The listing builds one solid part. Answer for the finished solid, in the listing's coordinates (mm). A direction names the side the tool comes from. Coordinates: 2 decimals unless noted, no trailing zeros. Order: outer loops, then holes, each group sorted by start corner. A loop starts at its lowest first (then second) coordinate and runs counter-clockwise, first axis right, second up. Notation, with made-up numbers: (45.25, 70) -> (98.25, 70) arc R16 cw to (98.25, 75) -> close; hole circle Ø8 at (39.5, 47.5). An arc over 180 degrees is marked (long way). Return JSON: item names as keys, results as strings.
Autodesk Inventor part; units mm, degrees
ref_plane "YZ Plane" through (0, 0, 0) normal (1, 0, 0) x (0, 1, 0)
ref_plane "XZ Plane" through (0, 0, 0) normal (0, 1, 0) x (-1, 0, 0)
ref_plane "XY Plane" through (0, 0, 0) normal (0, 0, 1) x (1, 0, 0)
sketch "スケッチ1" plane through (0, 0, 0) normal (0, 0, 1) x (1, 0, 0)
  circle A0 centre (-35.9404, 22.842) radius 1.5
  circle A1 centre (5.9362, 53.5882) radius 1.5
  circle A2 centre (127.6431, 30.2622) radius 1.5
  line L0 (22.1499, 50.4807) -> (113.9448, 32.8876)
  circle A3 centre (5.9362, 53.5882) radius 4.5
  circle A4 centre (127.6431, 30.2622) radius 4.5
  circle A5 centre (-35.9404, 22.842) radius 3
  line L1 (5.0892, 49.1686) -> (11.145, 48.008)
  line L2 (11.145, 48.008) -> (22.1499, 50.4807)
  line L3 (113.9448, 32.8876) -> (122.4523, 26.6751)
  line L4 (122.4523, 26.6751) -> (126.7961, 25.8426)
  line L5 (4.4419, 57.8328) -> (15.2047, 61.622)
  line L6 (-37.785, 25.2079) -> (3.1694, 57.1371)
  line L7 (3.5126, 49.7966) -> (-34.0959, 20.4761)
  line L8 (122.0018, 41.1536) -> (130.601, 33.6535)
  circle A6 centre (80.3181, 36.2778) radius 3
  circle A7 centre (80.3181, 36.2778) radius 4.5
  line L9 (128.2106, 34.7263) -> (80.8855, 40.7419)
  circle A8 centre (80.4743, 23.124) radius 1.5
  line L10 (120.4636, 35.711) -> (121.0283, 38.6574)
  line L11 (15.1864, 58.9428) -> (14.6217, 55.9964)
  circle A9 centre (66.9779, 42.9073) radius 1.5
  circle A10 centre (66.9779, 42.9073) radius 3
  line L12 (29.9182, 56.1193) -> (29.3535, 53.1729)
  arc A11 (17.2488, 58.5475) -> (15.1864, 58.9428) centre (16.2176, 58.7451) ccw
  arc A12 (29.9182, 56.1193) -> (27.8558, 56.5146) centre (28.887, 56.3169) ccw
  arc A13 (27.2911, 53.5682) -> (29.3535, 53.1729) centre (28.3223, 53.3705) ccw
  arc A14 (14.6217, 55.9964) -> (16.6841, 55.6011) centre (15.6529, 55.7987) ccw
  line L13 (17.2488, 58.5475) -> (27.8558, 56.5146)
  line L14 (16.6841, 55.6011) -> (27.2911, 53.5682)
  arc A15 (31.8825, 55.7428) -> (27.0019, 58.7146) centre (28.887, 56.3169) ccw
  line L15 (27.0019, 58.7146) -> (18.8556, 60.2759)
  arc A16 (18.8556, 60.2759) -> (15.2047, 61.622) centre (16.2176, 58.7451) ccw
  line L16 (106.2964, 41.4808) -> (105.7317, 38.5345)
  arc A17 (108.3589, 41.0856) -> (106.2964, 41.4808) centre (107.3276, 41.2832) ccw
  arc A18 (121.0283, 38.6574) -> (118.9658, 39.0527) centre (119.997, 38.855) ccw
  arc A19 (118.4011, 36.1063) -> (120.4636, 35.711) centre (119.4323, 35.9086) ccw
  arc A20 (105.7317, 38.5345) -> (107.7942, 38.1392) centre (106.7629, 38.3368) ccw
  line L17 (31.8825, 55.7428) -> (104.3322, 41.8573)
  line L18 (108.3589, 41.0856) -> (118.9658, 39.0527)
  line L19 (107.7942, 38.1392) -> (118.4011, 36.1063)
  arc A21 (122.0018, 41.1536) -> (118.1119, 41.2527) centre (119.997, 38.855) ccw
  line L20 (118.1119, 41.2527) -> (109.9656, 42.814)
  arc A22 (109.9656, 42.814) -> (104.3322, 41.8573) centre (107.3276, 41.2832) ccw
  line L21 (30.3885, 58.9717) -> (38.2584, 54.5208)
  line L22 (16.7917, 61.7406) -> (29.4611, 59.3124)
  line L23 (120.5711, 41.8505) -> (107.9017, 44.2787)
  line L24 (106.8479, 44.2952) -> (98.5267, 42.97)
  point P0 (0, 0)
  point P1 (0, 0)
  point P2 (0, 0)
  dimension "d53" = 9
  dimension "d49" = 9
  dimension "d50" = 9
  dimension "d51" = 6
  dimension "d52" = 6
  dimension "d54" = 47.7059
  dimension "d55" = 47.7059
  dimension "d56" = 3
  dimension "d57" = 3
  dimension "d58" = 8.0769
  dimension "d59" = 8.0769
  dimension "d60" = 3
  dimension "d61" = 6
  dimension "d62" = 61.9691
  dimension "d63" = 61.9691
  dimension "d64" = 15
  dimension "d65" = 2.1
  dimension "d66" = 2
  dimension "d67" = 2
  dimension "d68" = 2
  dimension "d69" = 15
  dimension "d70" = 2.1
  dimension "d71" = 7
  dimension "d72" = 2
  dimension "d73" = 2
sketch "スケッチ2" plane through (0, 0, 0) normal (0, 0, 1) x (1, 0, 0)
  line L0 (17.1, 0) -> (90.6683, 0)
  line L1 (107.7683, 0) -> (107.7683, -47)
  line L2 (90.6683, -47) -> (17.1, -47)
  line L3 (0, -47) -> (0, 0)
  line L4 (0, 0) -> (0, 3)
  line L5 (0, 3) -> (15, 3)
  line L6 (15, 3) -> (15, 0)
  line L7 (107.7683, 0) -> (107.7683, 3)
  line L8 (107.7683, 3) -> (92.7683, 3)
  line L9 (92.7683, 3) -> (92.7683, 0)
  line L10 (107.7683, -47) -> (107.7683, -50)
  line L11 (107.7683, -50) -> (92.7683, -50)
  line L12 (92.7683, -50) -> (92.7683, -47)
  line L13 (0, -47) -> (0, -50)
  line L14 (0, -50) -> (15, -50)
  line L15 (15, -50) -> (15, -47)
  arc A0 (15, 0) -> (17.1, 0) centre (16.05, 0) ccw
  arc A1 (90.6683, 0) -> (92.7683, 0) centre (91.7183, 0) ccw
  arc A2 (92.7683, -47) -> (90.6683, -47) centre (91.7183, -47) ccw
  arc A3 (17.1, -47) -> (15, -47) centre (16.05, -47) ccw
  line L16 (15.1864, 58.9428) -> (14.6217, 55.9964)
  line L17 (120.4636, 35.711) -> (121.0283, 38.6574)
  dimension "d30" = 107.7683
  dimension "d31" = 47
  dimension "d32" = 3
  dimension "d33" = 15
  dimension "d34" = 3
  dimension "d35" = 15
  dimension "d36" = 3
  dimension "d37" = 15
  dimension "d38" = 3
  dimension "d39" = 3
  dimension "d40" = 15
  dimension "d41" = 2.1
  dimension "d42" = 2.1
  dimension "d43" = 2.1
  dimension "d44" = 2.1
  dimension "d45" = 3
  dimension "d46" = 3
  dimension "d74" = 107.7683
extrude "押し出し1" add sketch "スケッチ2" along normal blind 3
sketch "スケッチ3" plane through (0, 0, 0) normal (0, 0, -1) x (-1, 0, 0)
  line L0 (0, 3) -> (0, -50)
  line L1 (-15, 3) -> (0, 3)
  line L2 (-15, 0) -> (-15, 3)
  arc A0 (-17.1, 0) -> (-15, 0) centre (-16.05, 0) ccw
  line L3 (-90.6683, 0) -> (-17.1, 0)
  arc A1 (-92.7683, 0) -> (-90.6683, 0) centre (-91.7183, 0) ccw
  line L4 (-92.7683, 3) -> (-92.7683, 0)
  line L5 (-107.7683, 3) -> (-92.7683, 3)
  line L6 (-107.7683, -50) -> (-107.7683, 3)
  line L7 (-92.7683, -50) -> (-107.7683, -50)
  line L8 (-92.7683, -47) -> (-92.7683, -50)
  arc A2 (-90.6683, -47) -> (-92.7683, -47) centre (-91.7183, -47) ccw
  line L9 (-17.1, -47) -> (-90.6683, -47)
  arc A3 (-15, -47) -> (-17.1, -47) centre (-16.05, -47) ccw
  line L10 (-15, -50) -> (-15, -47)
  line L11 (0, -50) -> (-15, -50)
  line L12 (-104.7683, -3) -> (-3, -3)
  line L13 (-3, -3) -> (-3, -44)
  line L14 (-3, -44) -> (-104.7683, -44)
  line L15 (-104.7683, -44) -> (-104.7683, -3)
  line L16 (-104.7683, -3) -> (-3, -44) construction
  arc A4 (-104.2078, -1.6087) -> (-106.2683, -3) centre (-104.7683, -3) ccw
  arc A5 (-3.5605, -45.3913) -> (-2.4395, -42.6087) centre (-3, -44) ccw
  line L17 (-3, -3) -> (-104.7683, -44) construction
  arc A6 (-2.4395, -4.3913) -> (-3.5605, -1.6087) centre (-3, -3) ccw
  arc A7 (-105.3288, -42.6087) -> (-104.2078, -45.3913) centre (-104.7683, -44) ccw
  line L18 (-3, -42.3828) -> (-49.8701, -23.5)
  line L19 (-53.8842, -21.8828) -> (-100.7543, -3)
  line L20 (-100.7543, -44) -> (-53.8842, -25.1172)
  line L21 (-49.8701, -23.5) -> (-3, -4.6172)
  line L22 (-104.7683, -4.6172) -> (-57.8982, -23.5)
  line L23 (-53.8842, -25.1172) -> (-7.014, -44)
  line L24 (-7.014, -3) -> (-53.8842, -21.8828)
  line L25 (-57.8982, -23.5) -> (-104.7683, -42.3828)
  point P0 (0, 0)
  point P1 (-53.8842, -23.5)
  point P2 (-53.8842, -23.5)
  dimension "d75" = 3
  dimension "d76" = 3
  dimension "d77" = 3
  dimension "d78" = 3
  dimension "d79" = 3
  dimension "d80" = 3
extrude "押し出し2" cut sketch "スケッチ3" against normal blind 2.5 contours L12 L24 L19 | L22 L25 L15 | L13 L18 L21 | L20 L23 L14
fillet "フィレット1" radius 1 12 edges at (100.7543, -3, 1.25) (104.7683, -4.6172, 1.25) (104.7683, -42.3828, 1.25) (100.7543, -44, 1.25) (57.8982, -23.5, 1.25) (53.8842, -21.8828, 1.25) (53.8842, -25.1172, 1.25) (49.8701, -23.5, 1.25) (7.014, -44, 1.25) (3, -42.3828, 1.25) (3, -4.6172, 1.25) (7.014, -3, 1.25)
equation "\"d55\" = d54"
equation "\"d59\" = d58"
equation "\"d63\" = d62"
equation "\"d30\" = d74"
properties part number "台形サスバー板" material "ポリカーボネート、クリア"
Item 1: Determine the mould class of faces 1 (the flat face through (92.768, 2, 1)), 2 (the cylindrical face through (91.7, -45.95, 1.48)), 3 (the flat face through (82.1, -13.75, 1.23)) for opening direction Y: pulls with the +Y half, pulls with the -Y half, needs draft (parallel to the pull), parting line crosses it, or undercut.
Answer list:
{"face 1": "needs draft", "face 2": "pulls with the -Y half", "face 3": "undercut"}
Item 2: Flat-ended cylindrical pins translate along their axes: pin 1 (1.5 mm diameter, centred on x = 60.5, z = 2, fed in from +Y); pin 2 (1.5 mm diameter, centred on x = 39.5, z = 2, fed in from -Y); pin 3 (5 mm diameter, centred on x = 65, y = -7, fed in from -Z). Find the tip coordinate at first contact, or state that the pin passes through.
Answer list:
{"pin 1": "y = 0", "pin 2": "y = -47", "pin 3": "z = 2.5"}
Item 3: Which of the six approach directions +Z, -Z, +X, -X, +Y, -Y give full straight-line access (tool end or side, diameter ignored) to faces 4 (the cylindrical face through (16.07, -1.05, 1.48)), 5 (the flat face through (15, -49, 1)), 6 (the cylindrical face through (11.187, -43.171, 1.268))?
Answer list:
{"face 4": "+Z, -Z, +Y", "face 5": "+Z, -Z, -Y", "face 6": "-Z"}
Item 4: The part is cut by section B-B on z = 1.05. Count the separate pieces of the cut face and the enclosed holes in it, plus the area to 3 significant figures.
Answer list:
{"separate pieces": "1", "enclosed holes": "4", "area": "1,720 mm2"}
Item 5: The part is cut by section D-D on x = 50.5. Determine the outline of the cut face in (y, z).
Answer list:
{"outline": "(-47, 0) -> (-44, 0) -> (-44, 2.5) -> (-26.48, 2.5) -> (-26.48, 0) -> (-20.52, 0) -> (-20.52, 2.5) -> (-3, 2.5) -> (-3, 0) -> (0, 0) -> (0, 3) -> (-47, 3) -> close"}
Item 6: The part is cut by section A-A on x = 16. Determine the outline of the cut face in (y, z).
Answer list:
{"outline": "(-45.95, 0) -> (-44, 0) -> (-44, 2.5) -> (-40.38, 2.5) -> (-40.38, 0) -> (-37.15, 0) -> (-37.15, 2.5) -> (-9.85, 2.5) -> (-9.85, 0) -> (-6.62, 0) -> (-6.62, 2.5) -> (-3, 2.5) -> (-3, 0) -> (-1.05, 0) -> (-1.05, 3) -> (-45.95, 3) -> close"}
Item 7: Find the intervals of material crossed by probe 1 along X at (y, z) = (-14, 1); probe 2 along Y at (x, z) = (58, 0.5); probe 3 along Y at (x, z) = (59, 0.95), in increasing order.
Answer list:
{"probe 1": "0 to 3, 26.29 to 34.32, 73.45 to 81.48, 104.77 to 107.77", "probe 2": "-47 to -44, -26.78 to -20.22, -3 to 0", "probe 3": "-47 to -44, -27.18 to -19.82, -3 to 0"}
Item 8: The part is cut by section C-C on y = -18. Determine the outline of the cut face in (x, z).
Answer list:
{"outline": "(0, 0) -> (3, 0) -> (3, 2.5) -> (36.22, 2.5) -> (36.22, 0) -> (44.25, 0) -> (44.25, 2.5) -> (63.52, 2.5) -> (63.52, 0) -> (71.55, 0) -> (71.55, 2.5) -> (104.77, 2.5) -> (104.77, 0) -> (107.77, 0) -> (107.77, 3) -> (0, 3) -> close"}
